Here's how the part is built. I have some questions about the finished solid (model axes, mm). A direction names the side the tool comes from. Give positions to 0.01 mm unless a question says otherwise; leave off trailing zeros. Write each loop counter-clockwise with the first axis right and the second up, starting at its lowest first coordinate (ties: lowest second). Pieces come first, ordered by that corner, then holes. Notation, with made-up numbers: (19, 48.5) -> (61, 48.5) arc R28 ccw to (61, 68.5) -> close; hole circle Ø8 at (37, -26). An arc over 180 degrees is marked (long way). Put each result on its own line as item: value. Start each with the question number.
from build123d import *

# Parameters (mm, degrees)
SKETCH1_4_W         = 15
SKETCH1_4_H         = 4
BOSS_EXTRUDE2_DEPTH = 7.5
CIRPATTERN1_COUNT   = 3


with BuildPart() as part:
    # Sketch1 → Revolve1 (revolve)
    with BuildSketch(Plane.YZ, mode=Mode.PRIVATE) as revolve1_sk:
        with BuildLine():
            Line((-107, 34.699971116), (-112, 34.699971116))
            Line((-112, 34.699971116), (-112, 30.699971116))
            Line((-112, 30.699971116), (-107.705307923, 30.699971116))
            Line((-107.705307923, 30.699971116), (-30.4, 2.563140081))
            Line((-30.4, 2.563140081), (-30.4, -19.471112681))
            ThreePointArc((-30.4, -19.471112681), (-45.908039104, -28.32676528), (-63.5, -31.4))
            Line((-63.5, -31.4), (-73.5, -31.4))
            ThreePointArc((-73.5, -31.4), (-82.5, -40.4), (-73.5, -49.4))
            Line((-73.5, -49.4), (-63.5, -49.4))
            Line((-63.5, -49.4), (-63.5, -45.4))
            Line((-63.5, -45.4), (-73.5, -45.4))
            ThreePointArc((-73.5, -45.4), (-78.5, -40.4), (-73.5, -35.4))
            Line((-73.5, -35.4), (-63.5, -35.4))
            ThreePointArc((-63.5, -35.4), (-46.370880058, -32.710274545), (-30.890538183, -24.9))
            ThreePointArc((-30.890538183, -24.9), (-28.073745645, -22.737267158), (-25.4, -20.4))
            Line((-25.4, -20.4), (-25.4, 5))
            Line((-25.4, 5), (-107, 34.699971116))
        make_face()
        with BuildLine():
            Line((-25.4, -24.9), (-25.4, -20.4))
            ThreePointArc((-25.4, -20.4), (-28.073745645, -22.737267158), (-30.890538183, -24.9))
            Line((-30.890538183, -24.9), (-25.4, -24.9))
        make_face()
    revolve(revolve1_sk.sketch.rotate(Axis((0, 0, 59.888434314), (0, 0, -1)), 270), axis=Axis((0, 0, 59.888434314), (0, 0, -1)))

    # Sketch1_4 → Boss-Extrude2 (add, symmetric)
    with BuildSketch(Plane.YZ):
        with BuildLine():
            Line((-73.5, -31.4), (-63.5, -31.4))
            ThreePointArc((-63.5, -31.4), (-45.908039104, -28.32676528), (-30.4, -19.471112681))
            Line((-30.4, -19.471112681), (-30.4, 2.563140081))
            Line((-30.4, 2.563140081), (-107.705307923, 30.699971116))
            Line((-107.705307923, 30.699971116), (-127, 30.699971116))
            Line((-127, 30.699971116), (-127, -49.4))
            Line((-127, -49.4), (-73.5, -49.4))
            ThreePointArc((-73.5, -49.4), (-82.5, -40.4), (-73.5, -31.4))
        make_face()
        with BuildLine():
            Line((-107, 34.699971116), (-112, 34.699971116))
            Line((-112, 34.699971116), (-112, 30.699971116))
            Line((-112, 30.699971116), (-107.705307923, 30.699971116))
            Line((-107.705307923, 30.699971116), (-30.4, 2.563140081))
            Line((-30.4, 2.563140081), (-30.4, -19.471112681))
            ThreePointArc((-30.4, -19.471112681), (-45.908039104, -28.32676528), (-63.5, -31.4))
            Line((-63.5, -31.4), (-73.5, -31.4))
            ThreePointArc((-73.5, -31.4), (-82.5, -40.4), (-73.5, -49.4))
            Line((-73.5, -49.4), (-63.5, -49.4))
            Line((-63.5, -49.4), (-63.5, -45.4))
            Line((-63.5, -45.4), (-73.5, -45.4))
            ThreePointArc((-73.5, -45.4), (-78.5, -40.4), (-73.5, -35.4))
            Line((-73.5, -35.4), (-63.5, -35.4))
            ThreePointArc((-63.5, -35.4), (-46.370880058, -32.710274545), (-30.890538183, -24.9))
            ThreePointArc((-30.890538183, -24.9), (-28.073745645, -22.737267158), (-25.4, -20.4))
            Line((-25.4, -20.4), (-25.4, 5))
            Line((-25.4, 5), (-107, 34.699971116))
        make_face()
        with Locations((-119.5, 32.699971116)):
            Rectangle(SKETCH1_4_W, SKETCH1_4_H)
    boss_extrude2 = extrude(amount=BOSS_EXTRUDE2_DEPTH, both=True)

    # CirPattern1: Boss-Extrude2 ×3 about axis
    cirpattern1_axis = Axis((0, 0, 0), (0, 0, 1))
    for i in range(1, CIRPATTERN1_COUNT):
        add(boss_extrude2.rotate(cirpattern1_axis, i * 360 / CIRPATTERN1_COUNT))


solid = part.part
1) I need wall thicknesses on probe 1 along Z at (x, y) = (-51.5, -51.5); probe 2 along Y at (x, z) = (0, -16); probe 3 along X at (y, z) = (-54.5, -15). Which ranges of each line are inside material? Lowest first, please.
2) Which directions (+Z, -Z, +X, -X, +Y, -Y) give clear straight access to the entire face, cutting with the end or side of a thin tool? Please do faces 4 (the flat face through (-7.5, -90, -7)), 5 (the flat face through (94, -55, 30.7)), 6 (the flat face through (-7, 25, -24.9)), 7 (the flat face through (-73.976, 51.371, -6.761)).
3) I want a section at C-C, the plane z = 14. Write out the boundary of the cut face in (x, y), and give its area (3 significant figures).
4) I want a section at B-B, the plane z = 26.5. Write out the boundary of the cut face in (x, y), and give its area (3 significant figures).
5) Thinking about a two-plate mould opening in Y: for faces 1 (the conical face through (-6.61, 29.78, 6.86)), 2 (the flat face through (-110.038, 63.409, -6.761)), 3 (the flat face through (0, -127, -7)), which applies, released by +Y, released by -Y, zero draft, split by the parting line, or undercut?
6) I'm going to push flat-ended pins straight in: pin 1 Ø2 at (y, z) = (48, 26) entering from +X; pin 2 Ø4 at (x, y) = (33, 20) entering from -Z; pin 3 Ø4 at (x, z) = (-72, 7.5) entering from +Y. Where does each tip first touch, or does it pass through?
Established:
1. probe 1: z = -49.4 to -45.4, -35.4 to -31.4, 18.01 to 22.26
1. probe 2: y = -127 to -25.4, 25.4 to 30.4
1. probe 3: x = -7.5 to 7.5
2. face 4: -X, -Y
2. face 5: -Z, +X
2. face 6: -Z
2. face 7: +Y
3. outline: (-113.74, 57) -> (-56.89, 24.19) arc R61.82 ccw to (-7.5, -61.37) -> (-7.5, -127) -> (7.5, -127) -> (7.5, -61.37) arc R61.82 ccw to (56.89, 24.19) -> (113.74, 57) -> (106.24, 70) -> (49.39, 37.18) arc R61.82 ccw to (-49.39, 37.18) -> (-106.24, 70) -> close; hole circle Ø100.25 at (0, 0)
3. area: 7,050 mm2
4. outline: (-113.74, 57) -> (-86.78, 41.44) arc R96.17 ccw to (-7.5, -95.87) -> (-7.5, -127) -> (7.5, -127) -> (7.5, -95.87) arc R96.17 ccw to (86.78, 41.44) -> (113.74, 57) -> (106.24, 70) -> (79.28, 54.43) arc R96.17 ccw to (-79.28, 54.43) -> (-106.24, 70) -> close; hole circle Ø168.94 at (0, 0)
4. area: 8,030 mm2
5. face 1: undercut
5. face 2: released by +Y
5. face 3: released by -Y
6. pin 1: stops at x = 99.87
6. pin 2: stops at z = -30.49
6. pin 3: stops at y = 51.38
